Geometry: final body of the model. Coordinates: model frame, mm. A direction names the side the tool comes from. Give positions to 0.01 mm unless a question says otherwise; leave off trailing zeros. Loops run counter-clockwise (first coordinate to the right, second up) from the corner with the lowest first, then second, coordinate; pieces in that order, holes last.
from build123d import *

# Parameters (mm, degrees)
SKETCH2_W           = 6.35
SKETCH2_H           = 5.08
SKETCH2_R           = 1.5875
BOSS_EXTRUDE1_DEPTH = 6.35
SKETCH3_R           = 1.5
CUT_EXTRUDE1_DEPTH  = 13.2322679
BOSS_EXTRUDE2_DEPTH = 4.7625


with BuildPart() as part:
    # Sketch2 → Boss-Extrude1 (new body)
    # profile 1 of 2: a face of its own
    with BuildSketch(Plane(origin=(0, 0, 0), x_dir=(0, 0, -1), z_dir=(1, 0, 0))):
        with Locations((-3.175, 2.54)):
            Rectangle(SKETCH2_W, SKETCH2_H)
    # profile 2 of 2: a face of its own
    with BuildSketch(Plane(origin=(0, 0, 0), x_dir=(0, 0, -1), z_dir=(1, 0, 0))):
        with BuildLine():
            Line((6.597804878, 5.08), (0, 5.08))
            Line((0, 5.08), (0, 0))
            Line((0, 0), (6.597804878, 0))
            ThreePointArc((6.597804878, 0), (9.137804878, 2.54), (6.597804878, 5.08))
        make_face()
        with Locations((6.597804878, 2.54)):
            Circle(SKETCH2_R, mode=Mode.SUBTRACT)
    boss_extrude1 = extrude(amount=BOSS_EXTRUDE1_DEPTH)

    # Sketch3 → Cut-Extrude1 (cut, through all)
    with BuildSketch(Plane(origin=(0, 5.08, 0), x_dir=(1, 0, 0), z_dir=(0, 1, 0))):
        with Locations(Location((3.175, 0, 0), (0, 0, 270))):
            Circle(SKETCH3_R)
    cut_extrude1 = extrude(amount=-CUT_EXTRUDE1_DEPTH, mode=Mode.SUBTRACT)

    # Sketch4 → Boss-Extrude2 (add)
    with BuildSketch(Plane(origin=(6.35, 0, 0), x_dir=(0, 0, -1), z_dir=(1, 0, 0))):
        Polygon((-6.35, 0), (1.517804878, 0), (1.517804878, 2.54), (1.517804878, 5.08), (-6.35, 5.08), align=None)
    extrude(amount=BOSS_EXTRUDE2_DEPTH)

    # Mirror1: Boss-Extrude1, Cut-Extrude1 across plane
    add(boss_extrude1.mirror(Plane(origin=(8.73125, 0, 0), x_dir=(0, 0, 1), z_dir=(1, 0, 0))))
    add(cut_extrude1.mirror(Plane(origin=(8.73125, 0, 0), x_dir=(0, 0, 1), z_dir=(1, 0, 0))), mode=Mode.SUBTRACT)


solid = part.part
Item 1: Set-up query: faces 4 (the face through (11.112, 3, -4)), 5 (the face through (9, 0, 0)). Return all of +Z, -Z, +X, -X, +Y, -Y with unobstructed straight access to the full face (end or side cutting, diameter ignored); none if empty.
Values follow:
face 4: -Z, +Y, -Y
face 5: +Z, -Z, +X, -X, -Y
Item 2: Section query A-A on x = 3.5. Give the number of separate pieces and of enclosed holes in the cut face, plus the area to 3 significant figures.
Values follow:
separate pieces: 2
enclosed holes: 1
area: 53.1 mm2
Item 3: Draft query along Z for faces 1 (the face through (9, 3, 6.35)), 2 (the face through (1.844, 2.576, 0.692)), 3 (the face through (17.462, 3, -1)). Return one class per face: +Z half, -Z half, draft (parallel to the pull), parting line (faces both ways), or undercut.
Values follow:
face 1: +Z half
face 2: undercut
face 3: draft
Item 4: Ray query, probe 1 along X at (y, z) = (3.95, 0) (1 decimal); probe 2 along X at (y, z) = (4.65, -3); probe 3 along Z at (x, y) = (3, 3.15). Return the intervals inside material, ascending.
Values follow:
probe 1: x = 0 to 1.7, 4.7 to 12.8, 15.8 to 17.5
probe 2: x = 0 to 6.35, 11.11 to 17.46
probe 3: z = -9.06 to -8.06, -5.13 to -1.49, 1.49 to 6.35
Item 5: Section query C-C on z = 0. Return loops of the section in (x, y) (1 decimal), plus the area to 3 significant figures.
Values follow:
outline: (0, 0) - (1.7, 0) - (1.7, 5.1) - (0, 5.1) - close; (4.7, 0) - (12.8, 0) - (12.8, 5.1) - (4.7, 5.1) - close; (15.8, 0) - (17.5, 0) - (17.5, 5.1) - (15.8, 5.1) - close
area: 58.2 mm2
